Read the model definition and answer for the solid it produces. Units are mm, in the model's axes. Coordinates: 2 decimals unless noted, no trailing zeros. Write each loop counter-clockwise with the first axis right and the second up, starting at its lowest first coordinate (ties: lowest second). Pieces come first, ordered by that corner, then holes.
(1) Straight lines are drawn through the part: line 1 along Y through (x, z) = (0, 3.5); line 2 along Y through (x, z) = (0, 12.25); line 3 along Z through (x, y) = (-7.5, 8). For each, find the intervals that lie inside material, in ascending order.
(2) The part is cut by section A-A, the plane x = 0. Determine the outline of the cut face in (y, z), and give its area (3 significant figures).
(3) The part is cut by section B-B, the plane z = 2.25. Determine the outline of the cut face in (x, y).
(4) The part is cut by section C-C, the plane y = 44.5. Determine the outline of the cut face in (x, z), and give its area (3 significant figures).
(5) The part is cut by section D-D, the plane y = 2. Determine the outline of the cut face in (x, z).
(6) Determine the mould class of faces 1 (the cylindrical face through (-1.73, 7.81, 4.93)), 2 (the cylindrical face through (5.77, 171.09, 10.04)), 3 (the flat face through (12.5, 79, 5)) for opening direction Y: pulls with the +Y half, pulls with the -Y half, needs draft (parallel to the pull), parting line crosses it, or undercut.
(7) Given pin 1 (4 mm diameter, centred on x = -5.5, z = 6.5, fed in from -Y); pin 2 (12 mm diameter, centred on x = 7, y = 117.5, fed in from +Z); pin 3 (13 mm diameter, centred on x = 0, y = 0, fed in from +Z); pin 4 (1.5 mm diameter, centred on x = -9.5, z = 4, fed in from +Y), each flat-ended and moving along its own axis, determine where each tip first touches the part or whether it passes through.
Autodesk Inventor part; units mm, degrees
sketch "Skizze5" plane through (0, 0, 0) normal (0, 0, 1) x (1, 0, 0)
  circle A0 centre (0, 0) radius 12.5
  circle A1 centre (0, 0) radius 8
  circle A2 centre (0, 160) radius 12.5
  circle A3 centre (0, 160) radius 8
  line L0 (0, 0) -> (0, 160) construction
  line L1 (-12.5, 0) -> (-12.5, 160)
  line L2 (12.5, 0) -> (12.5, 160)
  circle A4 centre (0, 80) radius 3
  dimension "d98" = 25
  dimension "d99" = 16
  dimension "d100" = 160
  dimension "d110" = 16
  dimension "d116" = 6
  dimension "d117" = 80
extrude "Extrusion8" add sketch "Skizze5" along normal blind 10 contours A0 | A0 L1 A2 L2 | A2 | A4
extrude "Extrusion12" add sketch "Skizze5" along normal blind 6.3 from surface at 10 contours A2
chamfer "Fase1" distance 0.5 angle 45 4 edges at (-12.5, 80, 0) (0, -12.5, 0) (12.5, 80, 0) (0, 172.5, 0)
equation "\"Anlaufscheibe_Thickness\" = 1"
equation "\"BaseFrame_InnerWidth\" = 83"
equation "\"Rillenkugellager_Flanschdicke\" = 1.1"
properties part number "ParallelSystem_ProximalPart_SupportLink" material "PBT-Kunststoff"
Computed:
1. line 1: y = -12.5 to -8, 8 to 152, 168 to 172.5
1. line 2: y = 147.5 to 152, 168 to 172.5
1. line 3: z = 0 to 10
2. outline: (-12.5, 0.5) - (-12, 0) - (-8, 0) - (-8, 10) - (-12.5, 10) - close; (8, 0) - (152, 0) - (152, 16.3) - (147.5, 16.3) - (147.5, 10) - (8, 10) - close; (168, 0) - (172, 0) - (172.5, 0.5) - (172.5, 16.3) - (168, 16.3) - close
2. area: 1,590 mm2
3. outline: (-12.5, 0) arc R12.5 ccw to (12.5, 0) - (12.5, 160) arc R12.5 ccw to (-12.5, 160) - close; hole circle Ø16 at (0, 0); hole circle Ø16 at (0, 160)
4. outline: (-12.5, 0.5) - (-12, 0) - (12, 0) - (12.5, 0.5) - (12.5, 10) - (-12.5, 10) - close
4. area: 250 mm2
5. outline: (-12.5, 0.5) - (-12, 0) - (-7.75, 0) - (-7.75, 10) - (-12.5, 10) - close; (7.75, 0) - (12, 0) - (12.5, 0.5) - (12.5, 10) - (7.75, 10) - close
6. face 1: undercut
6. face 2: parting line crosses it
6. face 3: needs draft
7. pin 1: stops at y = -12
7. pin 2: stops at z = 10
7. pin 3: passes through
7. pin 4: stops at y = 168.93
